The model under review builds one solid part; all positions refer to its coordinate system, in mm. Face numbers are marked on the shaded views. Coordinates: 2 decimals unless noted, no trailing zeros. Order: outer loops, then holes, each group sorted by start corner. A loop starts at its lowest first (then second) coordinate and runs counter-clockwise, first axis right, second up. Notation, with made-up numbers: M -16.75,12 L -11.75,12 A23 cw -11.75,46 Z; hole C 68.25,47 d1. An arc over 180 degrees is marked long. Answer as CSV lines item,"result". Start each with the question number.
Q1. Consider section A-A on x = 0. Write out the cut boundary in (y, z), and give its area (3 significant figures).
Q2. Consider section C-C on y = -5.25. Write out the cut boundary in (x, z), and give its area (3 significant figures).
Q3. Wall thickness on L1, parallel to Z at x = 1, y = -6; L2, parallel to Y at x = 0, z = 37; L3, parallel to X at y = -9.5, z = -13: over which ranges is each line inside the solid? List them lowest first. Write a range as [from, to].
Q4. For P1, Ø1, axis at x = 3, z = -28.5, coming from the -Y side; P2, Ø1.5, axis at x = -15.5, y = -8.5, coming from the -Z side; P3, Ø3, axis at x = 18, y = -8.5, coming from the -Z side; P4, Ø2, axis at x = 18, z = -19, coming from the -Y side, all flat-tipped, find the tip position at first contact; note any pin that passes through.
Q5. Consider section D-D on z = -19. State how many separate pieces and enclosed holes the cut face has, and give its area (3 significant figures).
Q6. The part is to be moulded in two halves that separate along Z. For the marked faces 1, 2 and 3, say which applies: +Z half, -Z half, draft (parallel to the pull), parting line (faces both ways), or undercut.
Q7. Consider section B-B on z = 0. Write out the cut boundary in (x, y), and give its area (3 significant figures).
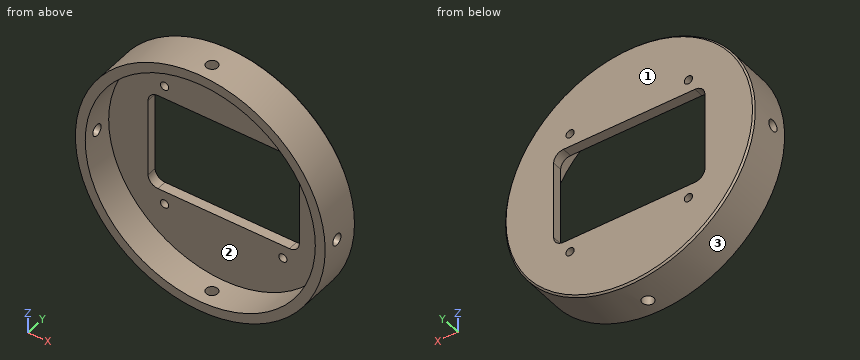
from build123d import *

# Parameters (mm, degrees)
F0_R     = 38
F1_DEPTH = 13
F2_T     = -3
F4_DEPTH = 25
F6_D     = 2.5
F9_D     = 3.5
F12_D    = 3.5
F13_SIZE = 0.5


with BuildPart() as f1:
    # F0 (on Front) → F1 (new body)
    with BuildSketch(Plane.XZ):
        Circle(F0_R)
    extrude(amount=F1_DEPTH)

    # F2
    f2_openings = [f1.faces().sort_by_distance(p)[0] for p in [
        (0, -13, 0),
    ]]
    offset(amount=F2_T, openings=f2_openings)

    # F3 (on face) → F4 (cut)
    with BuildSketch(Plane(origin=(0, 0, 0), x_dir=(-1, 0, 0), z_dir=(0, 1, 0))):
        with BuildLine():
            Line((20, 15), (-20, 15))
            ThreePointArc((-20, 15), (-22.1213203436, 14.1213203436), (-23, 12))
            Line((-23, 12), (-23, -12))
            ThreePointArc((-23, -12), (-22.1213203436, -14.1213203436), (-20, -15))
            Line((-20, -15), (20, -15))
            ThreePointArc((20, -15), (22.1213203436, -14.1213203436), (23, -12))
            Line((23, -12), (23, 12))
            ThreePointArc((23, 12), (22.1213203436, 14.1213203436), (20, 15))
        make_face()
    extrude(amount=-F4_DEPTH, mode=Mode.SUBTRACT)

    # F6 (through all)
    with Locations(Plane(origin=(0, 0, 0), x_dir=(-1, 0, 0), z_dir=(0, 1, 0))):
        with Locations((18, 19), (-18, 19), (-18, -19), (18, -19)):
            Hole(F6_D / 2)

    # F9 (through all)
    with Locations(Plane.YZ.offset(38)):
        with Locations((-8, 0)):
            Hole(F9_D / 2)

    # F12 (through all)
    with Locations(Plane.XY.offset(38)):
        with Locations((0, -8)):
            Hole(F12_D / 2)

    # F13
    f13_edges = [f1.edges().sort_by_distance(p)[0] for p in [
        (-38, 0, 0),
    ]]
    chamfer(f13_edges, length=F13_SIZE)


solid = f1.part
Evaluation:
1,outline,"M -13,-38 L -9.75,-38 L -9.75,-35 L -13,-35 Z; M -13,35 L -9.75,35 L -9.75,38 L -13,38 Z; M -6.25,-38 L -0.5,-38 L 0,-37.5 L 0,-15 L -3,-15 L -3,-35 L -6.25,-35 Z; M -6.25,35 L -3,35 L -3,15 L 0,15 L 0,37.5 L -0.5,38 L -6.25,38 Z"
1,area,"177 mm²"
2,outline,"C 0,0 d76; hole C 0,0 d70"
2,area,"688 mm²"
3,L1,"z = [-37.99, -34.99], [34.99, 37.99]"
3,L2,"y = [-13, -9.75], [-6.25, 0]"
3,L3,"x = [-35.71, -32.5], [32.5, 35.71]"
4,P1,"stops at y = -3"
4,P2,"stops at z = -35.02"
4,P3,"stops at z = -34.23"
4,P4,"passes through"
5,separate pieces,"3"
5,enclosed holes,"0"
5,area,"252 mm²"
6,face 1,"draft"
6,face 2,"undercut"
6,face 3,"parting line"
7,outline,"M -38,-13 L -35,-13 L -35,-9.75 L -38,-9.75 Z; M -38,-6.25 L -35,-6.25 L -35,-3 L -23,-3 L -23,0 L -37.5,0 L -38,-0.5 Z; M 23,-3 L 35,-3 L 35,-6.25 L 38,-6.25 L 38,-0.5 L 37.5,0 L 23,0 Z; M 35,-13 L 38,-13 L 38,-9.75 L 35,-9.75 Z"
7,area,"129 mm²"
